Check sheet for the drawn part. Datum: minimum x, y, z corner. Units: mm. Give positions to 0.01 mm unless a question says otherwise; leave off trailing zeros. Loops run counter-clockwise (first coordinate to the right, second up) from the corner with the lowest first, then second, coordinate; pieces in that order, holes last. Notation, with made-up numbers: (74.5, 3) - (122.5, 3) arc R17 cw to (122.5, 27) - close; hole circle Ø3 at (18, 18). An arc over 180 degrees is marked (long way). Answer in a Markdown table with one row per item.
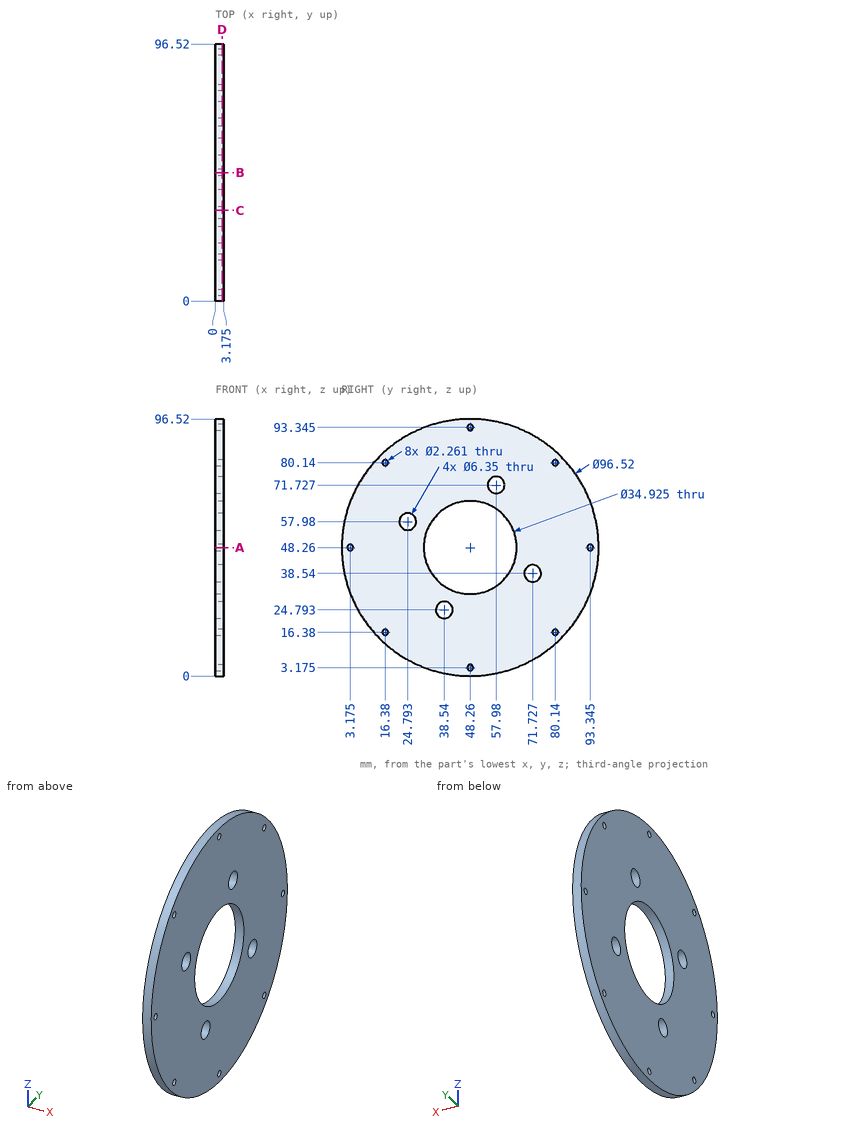
Q1. Thickness scan on line 1 (Y direction, x = 2.55, z = 48.26) (1 decimal); line 2 (Z direction, x = 0.8, y = 40.5) (1 decimal); line 3 (Y direction, x = 0.9, z = 59.5) (1 decimal). Record the ranges inside material, lowest first.
Completed:
| item | result |
|---|---|
| line 1 | 0 to 2, 4.3 to 30.8, 65.7 to 92.2, 94.5 to 96.5 |
| line 2 | 0.6 to 22.3, 27.3 to 32.6, 63.9 to 95.9 |
| line 3 | 1.3 to 22, 27.6 to 34.9, 61.6 to 95.2 |
Q2. Sectioned sample at D-D (x = 2.55). Give the number of separate pieces and of enclosed holes in the cut face, and give its area (3 significant figures).
Completed:
| item | result |
|---|---|
| separate pieces | 1 |
| enclosed holes | 13 |
| area | 6,200 mm^2 |
Q3. Sectioned sample at A-A (z = 48.26). Record the cut outline in (x, y) (1 decimal), and give its area (3 significant figures).
Completed:
| item | result |
|---|---|
| outline | (0, 0) - (3.2, 0) - (3.2, 2) - (0, 2) - close; (0, 4.3) - (3.2, 4.3) - (3.2, 30.8) - (0, 30.8) - close; (0, 65.7) - (3.2, 65.7) - (3.2, 92.2) - (0, 92.2) - close; (0, 94.5) - (3.2, 94.5) - (3.2, 96.5) - (0, 96.5) - close |
| area | 181 mm^2 |
Q4. Sectioned sample at C-C (y = 34). Record the cut outline in (x, z) (1 decimal).
Completed:
| item | result |
|---|---|
| outline | (0, 2.2) - (3.2, 2.2) - (3.2, 38.2) - (0, 38.2) - close; (0, 58.3) - (3.2, 58.3) - (3.2, 94.4) - (0, 94.4) - close |
